from build123d import *

# Parameters (mm, degrees)
F1_DEPTH  = 4
F3_DEPTH  = 2.5
F5_R      = 2.5
F6_DEPTH  = 2
F7_R      = 1.25
F8_DEPTH  = 4
F10_DEPTH = 2


with BuildPart() as f1:
    # F0 (on Right) → F1 (new body)
    with BuildSketch(Plane.YZ):
        with BuildLine():
            Line((0, 4), (0, 0))
            Line((0, 0), (8, 0))
            Line((8, 0), (8, 6))
            Line((8, 6), (16, 6))
            Line((16, 6), (16, 9))
            Line((16, 9), (8, 9))
            Line((8, 9), (8, 12))
            ThreePointArc((8, 12), (2.343146, 9.656854), (0, 4))
        make_face()
    extrude(amount=-F1_DEPTH)

    # F2 (on face) → F3 (cut)
    with BuildSketch(Plane.YZ):
        with BuildLine():
            Line((6.5, 0), (6.5, 10.324555))
            ThreePointArc((6.5, 10.324555), (2.90098, 8.031129), (1.5, 4))
            Line((1.5, 4), (1.5, 0))
            Line((1.5, 0), (6.5, 0))
        make_face()
    extrude(amount=-F3_DEPTH, mode=Mode.SUBTRACT)

    # F4: F1 across face


with BuildPart() as f1_1:
    add(f1.part)
    add(f1.part.mirror(Plane(origin=(0, 7.388969, 6.713356), x_dir=(0, 1, 0), z_dir=(1, 0, 0))))

    # F5 (on face) → F6 (join)
    with BuildSketch(Plane.XY.offset(9)):
        with Locations((0, 12)):
            Circle(F5_R)
    extrude(amount=F6_DEPTH)

    # F7 (on face) → F8 (cut)
    with BuildSketch(Plane(origin=(0, 0, 6), x_dir=(1, 0, 0), z_dir=(0, 0, -1))):
        with Locations((0, -12)):
            Circle(F7_R)
    extrude(amount=-F8_DEPTH, mode=Mode.SUBTRACT)

    # F9 (on face) → F10 (cut)
    with BuildSketch(Plane(origin=(0, 0, 6), x_dir=(1, 0, 0), z_dir=(0, 0, -1))):
        Polygon((-2.5, -8), (-2.5, -14.5), (2.5, -14.5), (2.5, -8), (0.5, -8), (0.5, -9.5), (-0.5, -9.5), (-0.5, -8), align=None)
    extrude(amount=-F10_DEPTH, mode=Mode.SUBTRACT)


solid = f1_1.part
Input: part model. Units: mm. Frame: model coordinates. A direction names the side the tool comes from. Coordinates: 2 decimals unless noted, no trailing zeros. Order: outer loops, then holes, each group sorted by start corner. A loop starts at its lowest first (then second) coordinate and runs counter-clockwise, first axis right, second up. Notation, with made-up numbers: M -6.5,32 L -2.5,32 A24 cw -2.5,64 Z; hole C 40,80.5 d9. An arc over 180 degrees is marked long. Answer in a Markdown table with one row per item.
(1) Material intervals for line 1 (X direction, y = 5, z = 4.5); line 2 (Y direction, x = 1, z = 7.5); line 3 (Y direction, x = 0, z = 9.4), sorted ascending. Write a range as [from, to].
Numbers:
| item | result |
|---|---|
| line 1 | x = [-4, -2.5], [2.5, 4] |
| line 2 | y = [0.81, 2.52], [6.5, 8], [14.5, 16] |
| line 3 | y = [2.1, 4.38], [6.5, 8], [9.5, 10.75], [13.25, 14.5] |
(2) Draft query along Y for faces 4 (the cylindrical face through (-0.54, 9.56, 9.99)), 5 (the flat face through (0, 9, 6)), 6 (the flat face through (0, 16, 7)). Return one class per face: pulls with the +Y half, pulls with the -Y half, needs draft (parallel to the pull), parting line crosses it, or undercut.
Numbers:
| item | result |
|---|---|
| face 4 | undercut |
| face 5 | needs draft |
| face 6 | pulls with the +Y half |
(3) Section query C-C, the plane x = 0. Output: boundary loops of the cut face in (y, z).
Numbers:
| item | result |
|---|---|
| outline | M 0,0 L 1.5,0 L 1.5,4 A6.5 cw 6.5,10.32 L 6.5,0 L 8,0 L 8,6 L 9.5,6 L 9.5,8 L 10.75,8 L 10.75,10 L 13.25,10 L 13.25,8 L 14.5,8 L 14.5,6 L 16,6 L 16,9 L 14.5,9 L 14.5,11 L 9.5,11 L 9.5,9 L 8,9 L 8,12 A8 ccw 0,4 Z |
(4) Contact query for flat-ended pins moving along their axis: pin 1 Ø4 at (x, z) = (-1.5, 8) entering from -Y; pin 2 Ø1.5 at (x, y) = (-1, 11) entering from -Z; pin 3 Ø2.5 at (x, y) = (-0.5, 12) entering from +Z. Output: stop coordinate, or through.
Numbers:
| item | result |
|---|---|
| pin 1 | stops at y = 0.25 |
| pin 2 | stops at z = 8 |
| pin 3 | stops at z = 11 |
(5) Access query for faces 1 (the flat face through (2.5, 11, 7)), 2 (the flat face through (0, 15, 6)), 3 (the flat face through (-2, 14, 9)). Directions: +Z, -Z, +X, -X, +Y, -Y. A direction counts if a zero-diameter tool reaches every point of the face in a straight line with its end or side. Return the directions, or none.
Numbers:
| item | result |
|---|---|
| face 1 | -Z |
| face 2 | -Z, +X, -X, +Y |
| face 3 | +Z |
(6) Section query A-A, the plane z = 3.75. Output: boundary loops of the cut face in (x, y), plus the area to 3 significant figures.
Numbers:
| item | result |
|---|---|
| outline | M -4,0 L 4,0 L 4,8 L -4,8 Z; hole M -2.5,1.5 L 2.5,1.5 L 2.5,6.5 L -2.5,6.5 Z |
| area | 39.0 mm^2 |
(7) Section query D-D, the plane z = 7. Output: boundary loops of the cut face in (x, y).
Numbers:
| item | result |
|---|---|
| outline | M -4,0.58 L 4,0.58 L 4,16 L -4,16 Z; hole M -2.5,2.23 L 2.5,2.23 L 2.5,6.5 L -2.5,6.5 Z; hole M -2.5,8 L -0.5,8 L -0.5,9.5 L 0.5,9.5 L 0.5,8 L 2.5,8 L 2.5,14.5 L -2.5,14.5 Z |
(8) Section query B-B, the plane y = 12. Output: boundary loops of the cut face in (x, z), plus the area to 3 significant figures.
Numbers:
| item | result |
|---|---|
| outline | M -4,6 L -2.5,6 L -2.5,8 L -1.25,8 L -1.25,10 L 1.25,10 L 1.25,8 L 2.5,8 L 2.5,6 L 4,6 L 4,9 L 2.5,9 L 2.5,11 L -2.5,11 L -2.5,9 L -4,9 Z |
| area | 19.0 mm^2 |
